from build123d import *

# Parameters (mm, degrees)
F0_W     = 40
F0_H     = 40
F1_DEPTH = 560
F3_D     = 8
F4_R     = 4


with BuildPart() as f1:
    # F0 (on Top) → F1 (new body)
    with BuildSketch(Plane.XY):
        Rectangle(F0_W, F0_H)
    extrude(amount=F1_DEPTH)

    # F3 (through all)
    with Locations(Plane.XY.offset(560)):
        with Locations((0, 0)):
            Hole(F3_D / 2)

    # F4
    f4_edges = [f1.edges().sort_by_distance(p)[0] for p in [
        (20, -20, 280),
        (-20, -20, 280),
        (20, 20, 280),
        (-20, 20, 280),
    ]]
    fillet(f4_edges, radius=F4_R)


solid = f1.part
Can you work these out from the model? Positions are in its coordinate system, mm. Round coordinates to 2 decimals unless told otherwise and drop trailing zeros. Loops run counter-clockwise (first coordinate to the right, second up) from the corner with the lowest first, then second, coordinate; pieces in that order, holes last. Notation, with made-up numbers: (45.5, 65) - (88.5, 65) arc R4 ccw to (88.5, 71) - close; hole circle Ø10 at (-36, 66). An arc over 180 degrees is marked (long way). Use CSV: the item, a comma, the result in double quotes. Start each with the question number.
1) For pin 1 Ø6 at (x, y) = (-3, -4) entering from -Z, with a flat end and sliding along its axis, tell me the tip position at first contact or that it passes through.
2) If we section it at A-A on z = 331: Write out the boundary of the cut face in (x, y).
3) Please list where these lines run through material, in increasing order: probe 1 along X at (y, z) = (0.5, 298); probe 2 along Y at (x, z) = (0, 270); probe 3 along Y at (x, z) = (-1.5, 515.5). Write a range as [from, to].
Geometry results:
1,pin 1,"stops at z = 0"
2,outline,"(-20, -16) arc R4 ccw to (-16, -20) - (16, -20) arc R4 ccw to (20, -16) - (20, 16) arc R4 ccw to (16, 20) - (-16, 20) arc R4 ccw to (-20, 16) - close; hole circle Ø8 at (0, 0)"
3,probe 1,"x = [-20, -3.97], [3.97, 20]"
3,probe 2,"y = [-20, -4], [4, 20]"
3,probe 3,"y = [-20, -3.71], [3.71, 20]"
